from build123d import *

# Parameters (mm, degrees)
BOSS_EXTRUDE1_DEPTH     = 1.52
SKETCH2_R               = 4.7625
CUT_EXTRUDE5_DEPTH      = 2.52
CUT_EXTRUDE5_DEPTH_BACK = 1


with BuildPart() as part:
    # Sketch1 → Boss-Extrude1 (new body)
    with BuildSketch(Plane(origin=(0, 0, 0), x_dir=(1, 0, 0), z_dir=(0, 1, 0))):
        with BuildLine():
            Line((-17.5, 30.310889132), (-17.5, 17.5))
            Line((-17.5, 17.5), (-30.310889132, 17.5))
            ThreePointArc((-30.310889132, 17.5), (-35, 0), (-30.310889132, -17.5))
            Line((-30.310889132, -17.5), (-17.5, -17.5))
            Line((-17.5, -17.5), (-17.5, -30.310889132))
            ThreePointArc((-17.5, -30.310889132), (0, -35), (17.5, -30.310889132))
            Line((17.5, -30.310889132), (17.5, -17.5))
            Line((17.5, -17.5), (30.310889132, -17.5))
            ThreePointArc((30.310889132, -17.5), (35, 0), (30.310889132, 17.5))
            Line((30.310889132, 17.5), (17.5, 17.5))
            Line((17.5, 17.5), (17.5, 30.310889132))
            ThreePointArc((17.5, 30.310889132), (0, 35), (-17.5, 30.310889132))
        make_face()
    extrude(amount=BOSS_EXTRUDE1_DEPTH)

    # Sketch2 → Cut-Extrude5 (cut, two sides)
    with BuildSketch(Plane(origin=(0, 0, 0), x_dir=(1, 0, 0), z_dir=(0, 1, 0))) as cut_extrude5_sk:
        Circle(SKETCH2_R)
        Polygon((-30.310889132, 17.5), (-17.5, 30.310889132), (-8.838834765, 8.838834765), align=None)
        Polygon((17.5, 30.310889132), (30.310889132, 17.5), (8.838834765, 8.838834765), align=None)
        Polygon((30.310889132, -17.5), (17.5, -30.310889132), (8.838834765, -8.838834765), align=None)
        Polygon((-30.310889132, -17.5), (-17.5, -30.310889132), (-8.838834765, -8.838834765), align=None)
    extrude(amount=CUT_EXTRUDE5_DEPTH, mode=Mode.SUBTRACT)
    extrude(cut_extrude5_sk.sketch, amount=-CUT_EXTRUDE5_DEPTH_BACK, mode=Mode.SUBTRACT)


solid = part.part
Can you work these out from the model? Positions are in its coordinate system, mm. A direction names the side the tool comes from. Give positions to 0.01 mm unless a question says otherwise; leave off trailing zeros. Loops run counter-clockwise (first coordinate to the right, second up) from the corner with the lowest first, then second, coordinate; pieces in that order, holes last. Notation, with made-up numbers: (32, 50.5) -> (71, 50.5) arc R14 ccw to (71, 58.5) -> close; hole circle Ø5 at (75.5, -40). An arc over 180 degrees is marked (long way). Use one line per item in the form item = value.
1) If we section it at C-C (y = 0.75): Please give me the cut outline in (x, z) (1 decimal), plus the area to 3 significant figures.
Answers:
outline = (-30.3, -17.5) -> (-8.8, -8.8) -> (-17.5, -30.3) arc R35 ccw to (17.5, -30.3) -> (8.8, -8.8) -> (30.3, -17.5) arc R35 ccw to (30.3, 17.5) -> (8.8, 8.8) -> (17.5, 30.3) arc R35 ccw to (-17.5, 30.3) -> (-8.8, 8.8) -> (-30.3, 17.5) arc R35 ccw to start; hole circle Ø9.5 at (0, 0)
area = 2,950 mm²
2) I need wall thicknesses on line 1 along X through (y, z) = (0.55, 13.5); line 2 along X through (y, z) = (0.4, 0); line 3 along X through (y, z) = (0.15, 9). Which ranges of each line are inside material? Lowest first, please.
Answers:
line_1 = -32.29 to -20.39, -10.72 to 10.72, 20.39 to 32.29
line_2 = -35 to -4.76, 4.76 to 35
line_3 = -33.82 to -9.24, -8.9 to 8.9, 9.24 to 33.82
3) If we section it at A-A (z = 0): Please give me the cut outline in (x, y), plus the area to 3 significant figures.
Answers:
outline = (-35, 0) -> (-4.76, 0) -> (-4.76, 1.52) -> (-35, 1.52) -> close; (4.76, 0) -> (35, 0) -> (35, 1.52) -> (4.76, 1.52) -> close
area = 91.9 mm²
4) If we section it at B-B (x = 0): Please give me the cut outline in (y, z), plus the area to 3 significant figures.
Answers:
outline = (0, -35) -> (1.52, -35) -> (1.52, -4.76) -> (0, -4.76) -> close; (0, 4.76) -> (1.52, 4.76) -> (1.52, 35) -> (0, 35) -> close
area = 91.9 mm²
5) We'd pull the mould along X, two halves only. Please class faces 1 (the face through (13.1, 0.7, -19.4)), 2 (the face through (35, 1, 0)), 3 (the face through (19.73, 0.75, -13.23)), 4 (the face through (0, 1.52, 7)): released by +X, released by -X, zero draft, split by the parting line, or undercut.
Answers:
face_1 = undercut
face_2 = released by +X
face_3 = undercut
face_4 = zero draft
6) If we section it at D-D (x = 11): Please give me the cut outline in (y, z), plus the area to 3 significant figures.
Answers:
outline = (0, -33.23) -> (1.52, -33.23) -> (1.52, -14.2) -> (0, -14.2) -> close; (0, -9.71) -> (1.52, -9.71) -> (1.52, 9.71) -> (0, 9.71) -> close; (0, 14.2) -> (1.52, 14.2) -> (1.52, 33.23) -> (0, 33.23) -> close
area = 87.4 mm²
7) For faces 5 (the face through (-35, 1, 0)), 6 (the face through (-13.23, 0.75, 19.73)), which set-ups out of +Z, -Z, +X, -X, +Y, -Y let a thin tool reach every point of the face, with its end or its side?
Answers:
face_5 = -X, +Y, -Y
face_6 = +Y, -Y
